from build123d import *

# Parameters (mm, degrees)
SKETCH1_W           = 25
SKETCH1_H           = 19
BOSS_EXTRUDE1_DEPTH = 7
SKETCH2_W           = 20
SKETCH2_H           = 15.5
CUT_EXTRUDE1_DEPTH  = 7
SKETCH4_R           = 2.5
CUT_EXTRUDE3_DEPTH  = 22.106870919
SKETCH5_R           = 2.5
CUT_EXTRUDE4_DEPTH  = 10


with BuildPart() as part:
    # Sketch1 → Boss-Extrude1 (new body)
    with BuildSketch(Plane.XY):
        Rectangle(SKETCH1_W, SKETCH1_H)
    extrude(amount=BOSS_EXTRUDE1_DEPTH)

    # Sketch2 → Cut-Extrude1 (cut)
    with BuildSketch(Plane.XY.offset(7)):
        with Locations((-2.5, 1.75)):
            Rectangle(SKETCH2_W, SKETCH2_H)
    extrude(amount=-CUT_EXTRUDE1_DEPTH, mode=Mode.SUBTRACT)

    # Sketch4 → Cut-Extrude3 (cut, through all)
    with BuildSketch(Plane(origin=(0, -6, 0), x_dir=(1, 0, 0), z_dir=(0, 1, 0))):
        with Locations(Location((0.5, -3.5, 0), (0, 0, 270))):
            Circle(SKETCH4_R)
    extrude(amount=-CUT_EXTRUDE3_DEPTH, mode=Mode.SUBTRACT)

    # Sketch5 → Cut-Extrude4 (cut)
    with BuildSketch(Plane(origin=(12.5, 0, 0), x_dir=(0, 0, -1), z_dir=(1, 0, 0))):
        with Locations(Location((-3.5, 5.5, 0), (0, 0, 90))):
            Circle(SKETCH5_R)
    extrude(amount=-CUT_EXTRUDE4_DEPTH, mode=Mode.SUBTRACT)


solid = part.part
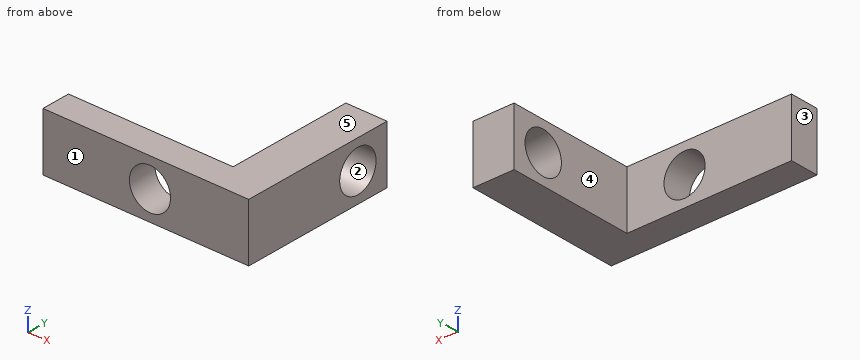
Part model, mm, in its own coordinate system. Face numbers are marked on the shaded views. A direction names the side the tool comes from. Give positions to 0.01 mm unless a question says otherwise; leave off trailing zeros. Order: outer loops, then holes, each group sorted by start corner. A loop starts at its lowest first (then second) coordinate and runs counter-clockwise, first axis right, second up. Notation, with made-up numbers: (82, 64.5) -> (138, 64.5) arc R26 cw to (138, 103.5) -> close; hole circle Ø11 at (4, 13.25). An arc over 180 degrees is marked (long way). Use one line per item in the form item = value.
(1) Drill centre lines: line 1 (X direction, y = -7.5, z = 3.5); line 2 (Z direction, x = 9.4, y = 5.5); line 3 (Y direction, x = -6.5, z = 5.75). Where is each one in solid material? Low to high. Write a range as from..to.
Solution:
line_1 = -12.5..-2, 3..12.5
line_2 = 0..1, 6..7
line_3 = -9.5..-6
(2) Saw through at B-B (z = 2). Write the cut outline in (x, y).
Solution:
outline = (-12.5, -9.5) -> (-1.5, -9.5) -> (-1.5, -6) -> (-12.5, -6) -> close; (2.5, -9.5) -> (12.5, -9.5) -> (12.5, 3.5) -> (7.5, 3.5) -> (7.5, -6) -> (2.5, -6) -> close; (7.5, 7.5) -> (12.5, 7.5) -> (12.5, 9.5) -> (7.5, 9.5) -> close
(3) Flat gauge pins, fed straight in: P1, Ø1, axis at x = 6, z = 1.5, coming from the +Y side; P2, Ø1.5, axis at y = 3.5, z = 3.5, coming from the +X side; P3, Ø1.5, axis at y = 7.5, z = 5, coming from the -X side. Where does each tip first touch, or does it go through?
Solution:
P1 = -6
P2 = 12.5
P3 = 7.5
(4) Saw through at D-D (y = -7). Write the cut outline in (x, z), then the cut area to 3 significant figures.
Solution:
outline = (-12.5, 0) -> (12.5, 0) -> (12.5, 7) -> (-12.5, 7) -> close; hole circle Ø5 at (0.5, 3.5)
area = 155 mm²
(5) Pull direction Y, two halves, no side cores. Call the marked faces 1, 2 and 3: +Y half, -Y half, draft (parallel to the pull), parting line (faces both ways), or undercut.
Solution:
face_1 = -Y half
face_2 = undercut
face_3 = draft
(6) Saw through at C-C (x = 0.5). Write the cut outline in (y, z), then the cut area to 3 significant figures.
Solution:
outline = (-9.5, 0) -> (-6, 0) -> (-6, 1) -> (-9.5, 1) -> close; (-9.5, 6) -> (-6, 6) -> (-6, 7) -> (-9.5, 7) -> close
area = 7.00 mm²
(7) Saw through at A-A (y = 5.5). Write the cut outline in (x, z).
Solution:
outline = (7.5, 0) -> (12.5, 0) -> (12.5, 1) -> (7.5, 1) -> close; (7.5, 6) -> (12.5, 6) -> (12.5, 7) -> (7.5, 7) -> close
(8) Tool access for the marked faces 4 and 5: list every direction of +Z, -Z, +X, -X, +Y, -Y with a clear straight run to the whole face (end or side of a thin tool).
Solution:
face_4 = +Z, -Z, -X, +Y
face_5 = +Z, +X, -X, +Y, -Y
